The model under review builds one solid part; all positions refer to its coordinate system, in mm. A direction names the side the tool comes from. Round coordinates to 2 decimals unless told otherwise and drop trailing zeros. Write each loop counter-clockwise with the first axis right and the second up, starting at its lowest first coordinate (ties: lowest second). Pieces come first, ordered by that corner, then holes. Notation, with made-up numbers: (-22, 41) - (-9, 41) arc R26 cw to (-9, 61) - close; hole circle Ø2 at (8.5, 76). An arc over 180 degrees is marked (long way). Use one line per item in the form item = value.
from build123d import *

# Parameters (mm, degrees)
BOSS_EXTRUDE1_DEPTH     = 20.95
BOSS_EXTRUDE2_DEPTH     = 2.75
SKETCH6_R               = 2
CUT_EXTRUDE2_DEPTH      = 10
CUT_EXTRUDE3_DEPTH      = 2.75
CUT_EXTRUDE4_DEPTH      = 39.517830206
CUT_EXTRUDE4_DEPTH_BACK = 39.517830206
SKETCH8_W               = 8.290514233
SKETCH8_H               = 3.25
CUT_EXTRUDE5_REACH      = 64.495
SKETCH9_W               = 12.1
SKETCH9_H               = 9.7


with BuildPart() as part:
    # Sketch2 → Boss-Extrude1 (new body)
    with BuildSketch(Plane.XY):
        with BuildLine():
            Line((-14.709485767, 8), (-23, 8))
            Line((-23, 8), (-23, -19.25))
            Line((-23, -19.25), (23, -19.25))
            Line((23, -19.25), (23, 8))
            Line((23, 8), (14.709485767, 8))
            ThreePointArc((14.709485767, 8), (0, 22.709485767), (-14.709485767, 8))
        make_face()
        with BuildLine():
            Line((-7.55, -13.758885964), (-7.55, -17.25))
            Line((-7.55, -17.25), (7.55, -17.25))
            Line((7.55, -17.25), (7.55, -13.758885964))
            Line((7.55, -13.758885964), (9.25, -13.758885964))
            Line((9.25, -13.758885964), (9.25, -10.839741694))
            ThreePointArc((9.25, -10.839741694), (0, 14.25), (-9.25, -10.839741694))
            Line((-9.25, -10.839741694), (-9.25, -13.758885964))
            Line((-9.25, -13.758885964), (-7.55, -13.758885964))
        make_face(mode=Mode.SUBTRACT)
    extrude(amount=BOSS_EXTRUDE1_DEPTH)

    # Sketch3 → Boss-Extrude2 (add)
    with BuildSketch(Plane.XY):
        with BuildLine():
            Line((-14.709485767, 8), (-23, 8))
            Line((-23, 8), (-23, -19.25))
            Line((-23, -19.25), (23, -19.25))
            Line((23, -19.25), (23, 8))
            Line((23, 8), (14.709485767, 8))
            ThreePointArc((14.709485767, 8), (0, 22.709485767), (-14.709485767, 8))
        make_face()
    extrude(amount=BOSS_EXTRUDE2_DEPTH)

    # Sketch6 → Cut-Extrude2 (cut)
    with BuildSketch(Plane.XY.offset(20.95)):
        with Locations((-17.5, 0)):
            Circle(SKETCH6_R)
        with Locations((17.5, 0)):
            Circle(SKETCH6_R)
    extrude(amount=-CUT_EXTRUDE2_DEPTH, mode=Mode.SUBTRACT)

    # Sketch7 → Cut-Extrude3 (cut)
    with BuildSketch(Plane.XY.offset(20.95)):
        with BuildLine():
            Line((-17.5, 3.75), (17.5, 3.75))
            ThreePointArc((17.5, 3.75), (21.25, 0), (17.5, -3.75))
            Line((17.5, -3.75), (-17.5, -3.75))
            ThreePointArc((-17.5, -3.75), (-21.25, 0), (-17.5, 3.75))
        make_face()
    extrude(amount=-CUT_EXTRUDE3_DEPTH, mode=Mode.SUBTRACT)

    # Sketch8 → Cut-Extrude4 (cut, two sides: drawn at the far end of the back side and taken through both)
    with BuildSketch(Plane.XY.offset(20.95).offset(-CUT_EXTRUDE4_DEPTH_BACK)):
        with Locations((-18.854742884, 6.375)):
            Rectangle(SKETCH8_W, SKETCH8_H)
        with Locations((18.854742884, 6.375)):
            Rectangle(SKETCH8_W, SKETCH8_H)
    extrude(amount=CUT_EXTRUDE4_DEPTH + CUT_EXTRUDE4_DEPTH_BACK, mode=Mode.SUBTRACT)

    # Sketch9 → Cut-Extrude5 (cut, up to next)
    with BuildSketch(Plane(origin=(0, -19.25, -19.25), x_dir=(-1, 0, 0), z_dir=(0, 1, 0)), mode=Mode.PRIVATE) as cut_extrude5_sk1:
        with Locations((0, 32.85)):
            Rectangle(SKETCH9_W, SKETCH9_H)
    cut_extrude5_tool1 = extrude(cut_extrude5_sk1.sketch, amount=CUT_EXTRUDE5_REACH, mode=Mode.PRIVATE) & part.part
    add(cut_extrude5_tool1.solids().sort_by_distance((0, -19.25, 13.6))[0], mode=Mode.SUBTRACT)


solid = part.part
(1) Add section C-C on z = 14.25. Write out the cut boundary in (x, y), then the cut area to 3 significant figures.
Geometry results:
outline = (-23, -19.25) - (-6.05, -19.25) - (-6.05, -17.25) - (-7.55, -17.25) - (-7.55, -13.76) - (-9.25, -13.76) - (-9.25, -10.84) arc R14.25 cw (long way) to (9.25, -10.84) - (9.25, -13.76) - (7.55, -13.76) - (7.55, -17.25) - (6.05, -17.25) - (6.05, -19.25) - (23, -19.25) - (23, 4.75) - (14.71, 4.75) - (14.71, 8) arc R14.71 ccw to (-14.71, 8) - (-14.71, 4.75) - (-23, 4.75) - close; hole circle Ø4 at (-17.5, 0); hole circle Ø4 at (17.5, 0)
area = 789 mm2
(2) The part is to be moulded in two halves that separate along X. For faces 1 (the flat face through (19, 4.75, 10)), 2 (the cylindrical face through (0.323, 22.706, 10.328)), 3 (the flat face through (0, -1, 2.75)), say which applies: +X half, -X half, draft (parallel to the pull), parting line (faces both ways), or undercut.
Geometry results:
face_1 = draft
face_2 = parting line
face_3 = undercut
(3) Machinability: for faces 4 (the flat face through (6.05, -18, 14)), 5 (the flat face through (9.25, -12, 12)), 6 (the flat face through (0, -19.25, 8)), which of the approach directions +Z, -Z, +X, -X, +Y, -Y give a long, thin tool a straight path to every point of the face, cutting with its end or side? Answer none if there is none.
Geometry results:
face_4 = -Y
face_5 = +Z
face_6 = +Z, -Z, +X, -X, -Y
(4) To check wall thickness, follow L1, parallel to Y at x = 17.5, z = 15.5; L2, parallel to X at y = -15.5, z = 15; L3, parallel to Y at x = 0, z = 7.5. State the ranges of each line that lie inside material, in increasing order.
Geometry results:
L1 = -19.25 to -2, 2 to 4.75
L2 = -23 to -7.55, 7.55 to 23
L3 = -19.25 to -17.25, 14.25 to 22.71
(5) Add section D-D on y = -11.5. Write out the cut boundary in (x, z), then the cut area to 3 significant figures.
Geometry results:
outline = (-23, 0) - (23, 0) - (23, 20.95) - (9.25, 20.95) - (9.25, 2.75) - (-9.25, 2.75) - (-9.25, 20.95) - (-23, 20.95) - close
area = 627 mm2
(6) Insertion check: P1, Ø3, axis at x = -9, y = -3, coming from the +Z side; P2, Ø4.5, axis at x = 3.5, z = 13, coming from the +Y side; P3, Ø3.5, axis at x = -17.5, y = 0, coming from the +Z side. Each pin has a flat end and moves straight along its axis. Give the tip position at first contact, or say it passes through.
Geometry results:
P1 = 2.75
P2 = 22.66
P3 = 10.95
(7) Add section A-A on x = 0. Write out the cut boundary in (y, z).
Geometry results:
outline = (-19.25, 0) - (22.71, 0) - (22.71, 20.95) - (14.25, 20.95) - (14.25, 2.75) - (-17.25, 2.75) - (-17.25, 8.75) - (-19.25, 8.75) - close; (-19.25, 18.45) - (-17.25, 18.45) - (-17.25, 20.95) - (-19.25, 20.95) - close
(8) Add section B-B on z = 19.5. Write out the cut boundary in (x, y).
Geometry results:
outline = (-23, -19.25) - (23, -19.25) - (23, 4.75) - (14.71, 4.75) - (14.71, 8) arc R14.71 ccw to (-14.71, 8) - (-14.71, 4.75) - (-23, 4.75) - close; hole (-17.5, -3.75) - (-13.75, -3.75) arc R14.25 ccw to (-9.25, -10.84) - (-9.25, -13.76) - (-7.55, -13.76) - (-7.55, -17.25) - (7.55, -17.25) - (7.55, -13.76) - (9.25, -13.76) - (9.25, -10.84) arc R14.25 ccw to (13.75, -3.75) - (17.5, -3.75) arc R3.75 ccw to (17.5, 3.75) - (13.75, 3.75) arc R14.25 ccw to (-13.75, 3.75) - (-17.5, 3.75) arc R3.75 ccw to start
